The figure shows three views and two pictorial views of one solid part (mm, origin at its lowest corner). Answer the questions. A direction names the side the tool comes from. Give positions to 0.01 mm unless a question says otherwise; leave off trailing zeros. Loops run counter-clockwise (first coordinate to the right, second up) from the corner with the lowest first, then second, coordinate; pieces in that order, holes last. Notation, with made-up numbers: (26, 25) - (30, 25) arc R15 cw to (30, 52) - close; hole circle Ø9 at (45.25, 44.25). An arc over 180 degrees is marked (long way). Write item = value, one per line.
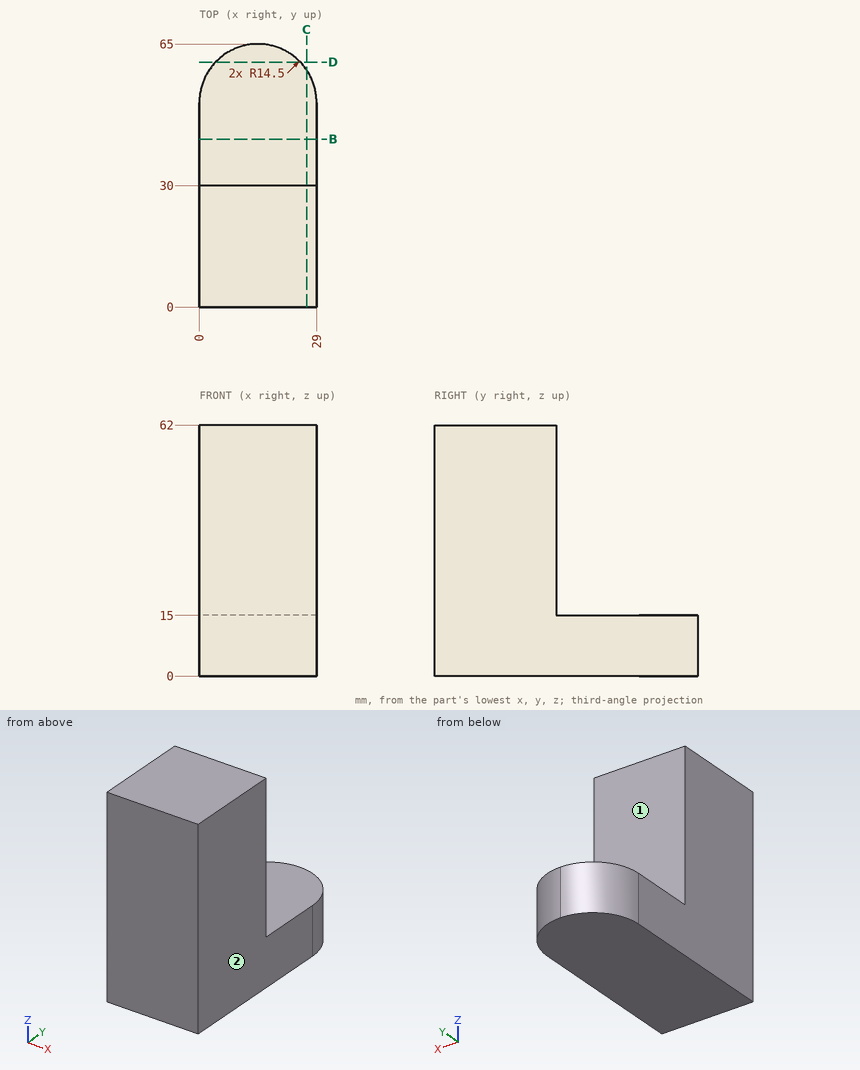
1) A cutting plane is placed at B-B on y = 41.5. Determine the outline of the cut face in (x, z).
Output:
outline = (0, 0) - (29, 0) - (29, 15) - (0, 15) - close
2) Find the intervals of material crossed by probe 1 along Z at (x, y) = (17.5, 42); probe 2 along Y at (x, z) = (17, 51); probe 3 along Y at (x, z) = (10.75, 8), in increasing order.
Output:
probe_1 = 0 to 15
probe_2 = 0 to 30
probe_3 = 0 to 64.51
3) Each of these flat-tipped pins is pushed along its axis until it touches: P1, Ø10, axis at x = 18.5, z = 25, coming from the +Y side; P2, Ø12, axis at x = 4.5, z = 10.5, coming from the +Y side; P3, Ø10, axis at x = 17.5, y = 55.5, coming from the +Z side. Where does it stop, or does it pass through?
Output:
P1 = 30
P2 = 64.44
P3 = 15
4) A tool of negligible diameter and unlimited length cuts with its end or side. For the marked faces 1 and 2, from which of +Z, -Z, +X, -X, +Y, -Y can it reach the whole face along a straight path? Write none if from no direction.
Output:
face_1 = +Z, +X, -X, +Y
face_2 = +Z, -Z, +X, +Y, -Y
5) A cutting plane is placed at C-C on x = 26.5. Determine the outline of the cut face in (y, z).
Output:
outline = (0, 0) - (58.64, 0) - (58.64, 15) - (30, 15) - (30, 62) - (0, 62) - close
6) A cutting plane is placed at D-D on y = 60.5. Determine the outline of the cut face in (x, z), then the cut area to 3 significant figures.
Output:
outline = (4, 0) - (25, 0) - (25, 15) - (4, 15) - close
area = 315 mm²
